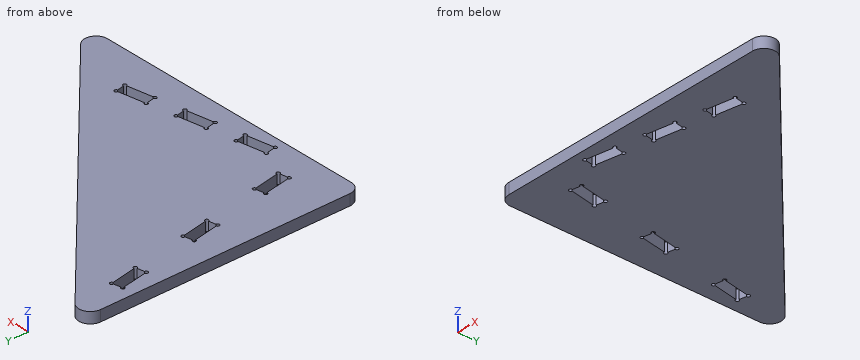
```python
from build123d import *

# Parameters (mm, degrees)
BOSS_EXTRUDE1_DEPTH = 19


with BuildPart() as part:
    # Sketch1 → Boss-Extrude1 (new body)
    with BuildSketch(Plane.XY):
        with BuildLine():
            Line((0, 20), (0, 454.788965914))
            ThreePointArc((0, 454.788965914), (11.908928303, 473.079251828), (33.45345588, 469.587767382))
            Line((33.45345588, 469.587767382), (511.721318385, 34.798801468))
            ThreePointArc((511.721318385, 34.798801468), (516.922299368, 12.788066464), (498.267862505, 0))
            Line((498.267862505, 0), (20, 0))
            ThreePointArc((20, 0), (5.857864376, 5.857864376), (0, 20))
        make_face()
        with BuildLine():
            Line((24.130575607, 397.736018906), (36.207010666, 400.074453065))
            ThreePointArc((36.207010666, 400.074453065), (40.847447332, 403.119941065), (39.685090804, 397.692457586))
            Line((39.685090804, 397.692457586), (47.499326679, 354.391906577))
            ThreePointArc((47.499326679, 354.391906577), (50.482851851, 349.709309806), (45.071751319, 350.953546922))
            Line((45.071751319, 350.953546922), (32.73690061, 348.928341259))
            ThreePointArc((32.73690061, 348.928341259), (28.041339197, 345.995030056), (29.255591906, 351.396715159))
            Line((29.255591906, 351.396715159), (21.706228811, 394.21128083))
            ThreePointArc((21.706228811, 394.21128083), (18.713515198, 398.865809266), (24.130575607, 397.736018906))
        make_face(mode=Mode.SUBTRACT)
        with BuildLine():
            Line((50.177802257, 250.014855954), (62.254237316, 252.353290113))
            ThreePointArc((62.254237316, 252.353290113), (66.894673982, 255.398778113), (65.732317454, 249.971294634))
            Line((65.732317454, 249.971294634), (73.546553329, 206.670743625))
            ThreePointArc((73.546553329, 206.670743625), (76.530078501, 201.988146855), (71.118977969, 203.23238397))
            Line((71.118977969, 203.23238397), (58.78412726, 201.207178307))
            ThreePointArc((58.78412726, 201.207178307), (54.088565847, 198.273867104), (55.302818556, 203.675552207))
            Line((55.302818556, 203.675552207), (47.753455461, 246.490117878))
            ThreePointArc((47.753455461, 246.490117878), (44.760741848, 251.144646314), (50.177802257, 250.014855954))
        make_face(mode=Mode.SUBTRACT)
        with BuildLine():
            Line((76.225028907, 102.293693002), (88.301463966, 104.632127162))
            ThreePointArc((88.301463966, 104.632127162), (92.941900632, 107.677615161), (91.779544104, 102.250131683))
            Line((91.779544104, 102.250131683), (99.59377998, 58.949580674))
            ThreePointArc((99.59377998, 58.949580674), (102.577305151, 54.266983903), (97.166204619, 55.511221018))
            Line((97.166204619, 55.511221018), (84.83135391, 53.486015355))
            ThreePointArc((84.83135391, 53.486015355), (80.135792497, 50.552704152), (81.350045206, 55.954389255))
            Line((81.350045206, 55.954389255), (73.800682111, 98.768954926))
            ThreePointArc((73.800682111, 98.768954926), (70.807968498, 103.423483362), (76.225028907, 102.293693002))
        make_face(mode=Mode.SUBTRACT)
        with BuildLine():
            Line((248.921064371, 52.485302628), (292.252605504, 60.125822445))
            ThreePointArc((292.252605504, 60.125822445), (296.927758072, 63.104223111), (295.727973296, 57.692343719))
            Line((295.727973296, 57.692343719), (297.898575517, 45.382246806))
            ThreePointArc((297.898575517, 45.382246806), (300.876976182, 40.707094238), (295.46509679, 41.906879014))
            Line((295.46509679, 41.906879014), (252.133555658, 34.266359197))
            ThreePointArc((252.133555658, 34.266359197), (247.45840309, 31.287958531), (248.658187866, 36.699837923))
            Line((248.658187866, 36.699837923), (246.487585645, 49.009934835))
            ThreePointArc((246.487585645, 49.009934835), (243.509184979, 53.685087404), (248.921064371, 52.485302628))
        make_face(mode=Mode.SUBTRACT)
        with BuildLine():
            Line((150.44028907, 35.120484861), (193.771830203, 42.761004678))
            ThreePointArc((193.771830203, 42.761004678), (198.446982771, 45.739405344), (197.247197995, 40.327525952))
            Line((197.247197995, 40.327525952), (199.417800215, 28.01742904))
            ThreePointArc((199.417800215, 28.01742904), (202.396200881, 23.342276471), (196.984321489, 24.542061247))
            Line((196.984321489, 24.542061247), (153.652780357, 16.90154143))
            ThreePointArc((153.652780357, 16.90154143), (148.977627789, 13.923140764), (150.177412565, 19.335020156))
            Line((150.177412565, 19.335020156), (148.006810344, 31.645117069))
            ThreePointArc((148.006810344, 31.645117069), (145.028409678, 36.320269637), (150.44028907, 35.120484861))
        make_face(mode=Mode.SUBTRACT)
        with BuildLine():
            Line((347.401839672, 69.850120394), (390.733380805, 77.490640212))
            ThreePointArc((390.733380805, 77.490640212), (395.408533373, 80.469040877), (394.208748597, 75.057161485))
            Line((394.208748597, 75.057161485), (396.379350818, 62.747064573))
            ThreePointArc((396.379350818, 62.747064573), (399.357751483, 58.071912005), (393.945872092, 59.271696781))
            Line((393.945872092, 59.271696781), (350.614330959, 51.631176963))
            ThreePointArc((350.614330959, 51.631176963), (345.939178391, 48.652776298), (347.138963167, 54.064655689))
            Line((347.138963167, 54.064655689), (344.968360946, 66.374752602))
            ThreePointArc((344.968360946, 66.374752602), (341.98996028, 71.04990517), (347.401839672, 69.850120394))
        make_face(mode=Mode.SUBTRACT)
    extrude(amount=BOSS_EXTRUDE1_DEPTH)


solid = part.part
```
Model file for the job. Use its own axes, mm. Give positions to 0.01 mm unless a question says otherwise; leave off trailing zeros. Write each loop counter-clockwise with the first axis right and the second up, starting at its lowest first coordinate (ties: lowest second). Pieces come first, ordered by that corner, then holes. Notation, with made-up numbers: (78, -27.5) - (85, -27.5) arc R16 ccw to (85, -14.5) - close; hole circle Ø8 at (79.5, 88). An arc over 180 degrees is marked (long way). One line per question, with ' | ' between items. Start each with the question number.
(1) Slice it at A-A on y = 360.5. Write the cut outline in (x, z), plus the area to 3 significant figures.
(2) Slice it at C-C on y = 235. Write the cut outline in (x, z), plus the area to 3 significant figures.
(3) Slice it at D-D on y = 160.5. Write the cut outline in (x, z).
(4) Pin check, flat tips, straight feed: P1, Ø3.5, axis at x = 48.03, y = 351.44, coming from the -Z side; P2, Ø10, axis at y = 139, z = 15, coming from the +X side; P3, Ø9.5, axis at x = 396.9, y = 59.79, coming from the -Z side; P4, Ø1, axis at y = 305.5, z = 3, coming from the +X side. Stop position of each tip, or through.
(5) Wall check: line 1 along X through (y, z) = (64.5, 5); line 2 along X through (y, z) = (34, 7); line 3 along Y through (x, z) = (377, 15.25). Give the ranges that are in metal, low to high. Write a range as from..to.
(6) Slice it at B-B on z = 7.75. Give the number of separate pieces and of enclosed holes in the cut face, plus the area to 3 significant figures.
Results below:
1) outline: (0, 0) - (27.65, 0) - (27.65, 19) - (0, 19) - close; (46.4, 0) - (153.45, 0) - (153.45, 19) - (46.4, 19) - close | area: 2,560 mm^2
2) outline: (0, 0) - (49.78, 0) - (49.78, 19) - (0, 19) - close; (68.43, 0) - (291.5, 0) - (291.5, 19) - (68.43, 19) - close | area: 5,180 mm^2
3) outline: (0, 0) - (373.45, 0) - (373.45, 19) - (0, 19) - close
4) P1: through | P2: x = 402.6 | P3: z = 0 | P4: x = 214.5
5) line 1: 0..79.84, 98.59..345.3, 396.07..479.05 | line 2: 0..144.55, 198.36..246.19, 252.17..512.55 | line 3: 0..56.28, 75.07..157.27
6) separate pieces: 1 | enclosed holes: 6 | area: 130,000 mm^2
